Input: part model. Units: mm. Frame: model coordinates. Coordinates: 2 decimals unless noted, no trailing zeros. Order: outer loops, then holes, each group sorted by start corner. A loop starts at its lowest first (then second) coordinate and runs counter-clockwise, first axis right, second up. Notation, with made-up numbers: M 0.5,36.5 L 44.5,36.5 A34 cw 44.5,74.5 Z; hole C 50,36.5 d3. An arc over 180 degrees is marked long. One line per item, written item: value.
```python
from build123d import *

# Parameters (mm, degrees)
BOSS_EXTRUDE1_DEPTH = 1.5875
SKETCH2_R           = 1.2446
CUT_EXTRUDE1_DEPTH  = 73.874128278
CUT_EXTRUDE2_DEPTH  = 3.175
SKETCH4_W           = 10.5156
SKETCH4_H           = 10.5156
SKETCH4_W_2         = 3.0734
SKETCH4_H_2         = 66.2432
SKETCH4_H_3         = 10.7442
CUT_EXTRUDE3_DEPTH  = 3.175
SKETCH5_W           = 21.1074
SKETCH5_H           = 2.8956
SKETCH5_H_2         = 5.4102
CUT_EXTRUDE4_DEPTH  = 3.175
SKETCH7_W           = 31.9532
SKETCH7_H           = 3.0734
CUT_EXTRUDE5_DEPTH  = 3.175
FILLET1_R           = 4.445
BOSS_EXTRUDE2_DEPTH = 3.175
BOSS_EXTRUDE3_DEPTH = 3.175


with BuildPart() as part:
    # Sketch1 → Boss-Extrude1 (new, symmetric)
    with BuildSketch(Plane(origin=(0, 0, 0), x_dir=(1, 0, 0), z_dir=(0, 1, 0))):
        Polygon((-20.2692, 48.5775), (-20.2692, 40.6527), (1.3208, 40.6527), (1.3208, 48.5775), (36.2966, 48.5775), (36.2966, 43.0657), (37.1348, 43.0657), (37.1348, 38.7223), (47.1424, 38.7223), (47.1424, 42.701382431), (44.1706, 42.701382431), (44.1706, 48.5775), (54.229, 48.5775), (54.229, -48.5775), (-54.229, -48.5775), (-54.229, 48.5775), align=None)
    extrude(amount=BOSS_EXTRUDE1_DEPTH, both=True)

    # Sketch2 → Cut-Extrude1 (cut, through all)
    with BuildSketch(Plane(origin=(0, 1.5875, 0), x_dir=(1, 0, 0), z_dir=(0, 1, 0))):
        with Locations(Location((-40.9956, 34.6837, 0), (0, 0, 270))):
            Circle(SKETCH2_R)
        with Locations(Location((-40.9956, -26.3271, 0), (0, 0, 270))):
            Circle(SKETCH2_R)
        with Locations(Location((40.9956, -26.3271, 0), (0, 0, 90))):
            Circle(SKETCH2_R)
        with Locations(Location((40.9956, 34.6837, 0), (0, 0, 90))):
            Circle(SKETCH2_R)
    extrude(amount=-CUT_EXTRUDE1_DEPTH, mode=Mode.SUBTRACT)

    # Sketch3 → Cut-Extrude2 (cut)
    with BuildSketch(Plane(origin=(0, 1.5875, 0), x_dir=(1, 0, 0), z_dir=(0, 1, 0))):
        with BuildLine():
            Line((-21.9456, 35.9283), (4.650175487, 35.9283))
            ThreePointArc((4.650175487, 35.9283), (5.599614823, 36.112421194), (6.41140699, 36.63809138))
            Line((6.41140699, 36.63809138), (6.842452629, 37.052891721))
            ThreePointArc((6.842452629, 37.052891721), (8.881692758, 43.876586936), (10.477108356, 36.935696088))
            Line((10.477108356, 36.935696088), (10.786368497, 36.63809138))
            ThreePointArc((10.786368497, 36.63809138), (11.598160664, 36.112421194), (12.5476, 35.9283))
            Line((12.5476, 35.9283), (27.0256, 35.9283))
            ThreePointArc((27.0256, 35.9283), (27.923625612, 35.556325612), (28.2956, 34.6583))
            Line((28.2956, 34.6583), (28.2956, 28.3337))
            ThreePointArc((28.2956, 28.3337), (28.667574388, 27.435674388), (29.5656, 27.0637))
            Line((29.5656, 27.0637), (32.1056, 27.0637))
            ThreePointArc((32.1056, 27.0637), (33.003625612, 26.691725612), (33.3756, 25.7937))
            Line((33.3756, 25.7937), (33.3756, 10.5029))
            ThreePointArc((33.3756, 10.5029), (33.003625612, 9.604874388), (32.1056, 9.2329))
            Line((32.1056, 9.2329), (28.2956, 9.2329))
            ThreePointArc((28.2956, 9.2329), (27.397574388, 8.860925612), (27.0256, 7.9629))
            Line((27.0256, 7.9629), (27.0256, -12.3571))
            ThreePointArc((27.0256, -12.3571), (26.653625612, -13.255125612), (25.7556, -13.6271))
            Line((25.7556, -13.6271), (19.4056, -13.6271))
            ThreePointArc((19.4056, -13.6271), (18.507574388, -13.999074388), (18.1356, -14.8971))
            Line((18.1356, -14.8971), (18.1356, -26.3271))
            ThreePointArc((18.1356, -26.3271), (17.763625612, -27.225125612), (16.8656, -27.5971))
            Line((16.8656, -27.5971), (-16.8656, -27.5971))
            ThreePointArc((-16.8656, -27.5971), (-17.763625612, -27.225125612), (-18.1356, -26.3271))
            Line((-18.1356, -26.3271), (-18.1356, -19.9771))
            ThreePointArc((-18.1356, -19.9771), (-18.507574388, -19.079074388), (-19.4056, -18.7071))
            Line((-19.4056, -18.7071), (-37.1856, -18.7071))
            ThreePointArc((-37.1856, -18.7071), (-38.083625612, -18.335125612), (-38.4556, -17.4371))
            Line((-38.4556, -17.4371), (-38.4556, -7.2771))
            ThreePointArc((-38.4556, -7.2771), (-38.083625612, -6.379074388), (-37.1856, -6.0071))
            Line((-37.1856, -6.0071), (-35.9156, -6.0071))
            ThreePointArc((-35.9156, -6.0071), (-35.017574388, -5.635125612), (-34.6456, -4.7371))
            Line((-34.6456, -4.7371), (-34.6456, 0.3429))
            ThreePointArc((-34.6456, 0.3429), (-34.273625612, 1.240925612), (-33.3756, 1.6129))
            Line((-33.3756, 1.6129), (-24.4856, 1.6129))
            ThreePointArc((-24.4856, 1.6129), (-23.587574388, 1.984874388), (-23.2156, 2.8829))
            Line((-23.2156, 2.8829), (-23.2156, 34.6583))
            ThreePointArc((-23.2156, 34.6583), (-22.843625612, 35.556325612), (-21.9456, 35.9283))
        make_face()
    extrude(amount=-CUT_EXTRUDE2_DEPTH, mode=Mode.SUBTRACT)

    # Sketch4 → Cut-Extrude3 (cut)
    with BuildSketch(Plane(origin=(0, 1.5875, 0), x_dir=(1, 0, 0), z_dir=(0, 1, 0))):
        with Locations((28.6258, 42.3799)):
            Rectangle(SKETCH4_W, SKETCH4_H)
        with Locations((-50.5841, 8.5725)):
            Rectangle(SKETCH4_W_2, SKETCH4_H_2)
        with Locations((-50.5841, -35.687)):
            Rectangle(SKETCH4_W_2, SKETCH4_H_3)
        with Locations((50.4571, 8.5725)):
            Rectangle(SKETCH4_W_2, SKETCH4_H_2)
        with Locations((50.4571, -35.687)):
            Rectangle(SKETCH4_W_2, SKETCH4_H_3)
    extrude(amount=-CUT_EXTRUDE3_DEPTH, mode=Mode.SUBTRACT)

    # Sketch5 → Cut-Extrude4 (cut)
    with BuildSketch(Plane(origin=(0, 1.5875, 0), x_dir=(1, 0, 0), z_dir=(0, 1, 0))):
        with Locations((-34.6583, -31.4325)):
            Rectangle(SKETCH5_W, SKETCH5_H)
        with Locations((-34.6583, -37.7698)):
            Rectangle(SKETCH5_W, SKETCH5_H_2)
        with Locations((-11.5443, -37.7698)):
            Rectangle(SKETCH5_W, SKETCH5_H_2)
        with Locations((-11.5443, -31.4325)):
            Rectangle(SKETCH5_W, SKETCH5_H)
        with Locations((11.5697, -31.4325)):
            Rectangle(SKETCH5_W, SKETCH5_H)
        with Locations((11.5697, -37.7698)):
            Rectangle(SKETCH5_W, SKETCH5_H_2)
        with Locations((34.6837, -37.7698)):
            Rectangle(SKETCH5_W, SKETCH5_H_2)
        with Locations((34.6837, -31.4325)):
            Rectangle(SKETCH5_W, SKETCH5_H)
    extrude(amount=-CUT_EXTRUDE4_DEPTH, mode=Mode.SUBTRACT)

    # Sketch7 → Cut-Extrude5 (cut)
    with BuildSketch(Plane(origin=(0, 1.5875, 0), x_dir=(1, 0, 0), z_dir=(0, 1, 0))):
        with Locations((-25.654, -44.691406541)):
            Rectangle(SKETCH7_W, SKETCH7_H)
        with Locations((25.654, -44.590951919)):
            Rectangle(SKETCH7_W, SKETCH7_H)
    extrude(amount=-CUT_EXTRUDE5_DEPTH, mode=Mode.SUBTRACT)

    # Fillet1
    fillet1_edges = [part.edges().sort_by_distance(p)[0] for p in [
        (-54.229, 0, -48.5775),
        (54.229, 0, -48.5775),
        (54.229, 0, 48.5775),
        (-54.229, 0, 48.5775),
    ]]
    fillet(fillet1_edges, radius=FILLET1_R)

    # Sketch8 → Boss-Extrude2 (add)
    with BuildSketch(Plane(origin=(0, 1.5875, 0), x_dir=(1, 0, 0), z_dir=(0, 1, 0))):
        Polygon((37.1348, 43.0657), (37.1348, 38.7223), (47.1424, 38.7223), (47.1424, 43.0657), (47.1424, 43.7007), (36.2966, 43.7007), (36.2966, 43.0657), align=None)
    extrude(amount=-BOSS_EXTRUDE2_DEPTH)

    # Sketch9 → Boss-Extrude3 (add)
    with BuildSketch(Plane(origin=(0, 1.5875, 0), x_dir=(1, 0, 0), z_dir=(0, 1, 0))):
        Polygon((-23.2156, 34.6583), (-23.2156, 35.9283), (4.650175487, 35.9283), (4.650175487, 32.7533), (-23.2156, 32.7533), align=None)
        Polygon((28.2956, 34.6583), (28.2956, 35.9283), (12.5476, 35.9283), (12.5476, 32.7533), (28.2956, 32.7533), align=None)
    extrude(amount=-BOSS_EXTRUDE3_DEPTH)


solid = part.part
```
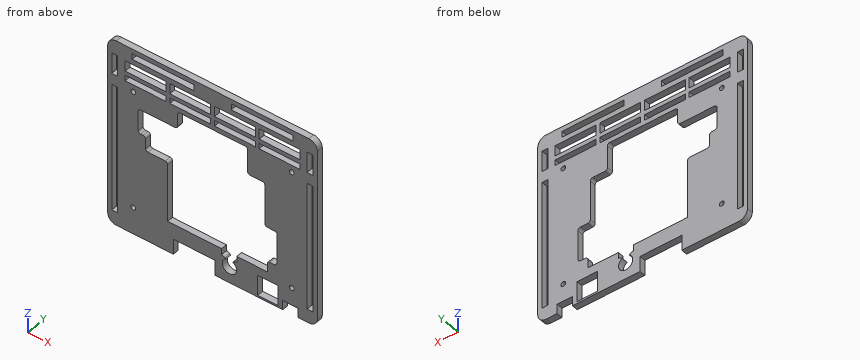
(1) Ray query, line 1 (X direction, y = -0.75, z = -20); line 2 (X direction, y = -0.8, z = 22); line 3 (Z direction, x = -16, y = -1.4). Return the intervals inside material, ascending. Write a range as from..to.
Data:
line 1: x = -54.23..-52.12, -49.05..-23.22, 33.38..48.92, 51.99..54.23
line 2: x = -54.23..-52.12, -49.05..-18.14, 18.14..48.92, 51.99..54.23
line 3: z = -40.65..-32.75, 27.6..29.98, 32.88..35.06, 40.47..43.15, 46.23..48.58
(2) Cut plane A-A on x = -14.5. Output: boundary loops of the cut face in (y, z).
Data:
outline: M -1.59,-40.65 L 1.59,-40.65 L 1.59,-32.75 L -1.59,-32.75 Z; M -1.59,27.6 L 1.59,27.6 L 1.59,29.98 L -1.59,29.98 Z; M -1.59,32.88 L 1.59,32.88 L 1.59,35.06 L -1.59,35.06 Z; M -1.59,40.47 L 1.59,40.47 L 1.59,43.15 L -1.59,43.15 Z; M -1.59,46.23 L 1.59,46.23 L 1.59,48.58 L -1.59,48.58 Z
(3) First-contact query: pin 1 (0.9 mm diameter, centred on x = -50.5, y = 0, fed in from -Z). Flat tip, straight axial feed; report the tip coordinate or a pass-through.
Data:
pin 1: stops at z = -48.57
(4) Cut plane B-B on z = -31. Output: boundary loops of the cut face in (x, y).
Data:
outline: M -54.23,-1.59 L -52.12,-1.59 L -52.12,1.59 L -54.23,1.59 Z; M -49.05,-1.59 L -23.22,-1.59 L -23.22,1.59 L -49.05,1.59 Z; M 28.3,-1.59 L 48.92,-1.59 L 48.92,1.59 L 28.3,1.59 Z; M 51.99,-1.59 L 54.23,-1.59 L 54.23,1.59 L 51.99,1.59 Z
(5) Cut plane C-C on z = -12.5. Output: boundary loops of the cut face in (x, y), plus the area to 3 significant figures.
Data:
outline: M -54.23,-1.59 L -52.12,-1.59 L -52.12,1.59 L -54.23,1.59 Z; M -49.05,-1.59 L -23.22,-1.59 L -23.22,1.59 L -49.05,1.59 Z; M 33.38,-1.59 L 48.92,-1.59 L 48.92,1.59 L 33.38,1.59 Z; M 51.99,-1.59 L 54.23,-1.59 L 54.23,1.59 L 51.99,1.59 Z
area: 145 mm2
(6) Cut plane D-D on y = 0.05. Give the number of separate pieces and of enclosed holes in the cut face, plus the area to 3 significant figures.
Data:
separate pieces: 1
enclosed holes: 20
area: 5,470 mm2
